```python
from build123d import *

# Parameters (mm, degrees)
BOSS_EXTRUDE1_DEPTH = 30
SKETCH2_R           = 2.25
CUT_EXTRUDE1_DEPTH  = 30
CUT_EXTRUDE2_DEPTH  = 30
CHAMFER1_SIZE       = 5


with BuildPart() as part:
    # Sketch1 → Boss-Extrude1 (new body)
    with BuildSketch(Plane.XY):
        Polygon((0, 22), (0, 0), (45, 0), (45, -3), (-3, -3), (-3, 22), align=None)
    extrude(amount=BOSS_EXTRUDE1_DEPTH)

    # Sketch2 → Cut-Extrude1 (cut)
    with BuildSketch(Plane(origin=(0, 0, 0), x_dir=(0, 0, -1), z_dir=(1, 0, 0))):
        with Locations(Location((-15, 12, 0), (0, 0, 90))):
            Circle(SKETCH2_R)
    extrude(amount=-CUT_EXTRUDE1_DEPTH, mode=Mode.SUBTRACT)

    # Sketch3 → Cut-Extrude2 (cut)
    with BuildSketch(Plane(origin=(0, 0, 0), x_dir=(1, 0, 0), z_dir=(0, 1, 0))):
        with BuildLine():
            Line((7.5, -13.25), (10.5, -13.25))
            ThreePointArc((10.5, -13.25), (12.25, -15), (10.5, -16.75))
            Line((10.5, -16.75), (7.5, -16.75))
            ThreePointArc((7.5, -16.75), (5.75, -15), (7.5, -13.25))
        make_face()
        with BuildLine():
            Line((32.5, -13.25), (35.5, -13.25))
            ThreePointArc((35.5, -13.25), (37.25, -15), (35.5, -16.75))
            Line((35.5, -16.75), (32.5, -16.75))
            ThreePointArc((32.5, -16.75), (30.75, -15), (32.5, -13.25))
        make_face()
    extrude(amount=-CUT_EXTRUDE2_DEPTH, mode=Mode.SUBTRACT)

    # Chamfer1
    chamfer1_edges = [part.edges().sort_by_distance(p)[0] for p in [
        (45, -1.5, 30),
        (-1.5, 22, 30),
        (45, -1.5, 0),
        (-1.5, 22, 0),
    ]]
    chamfer(chamfer1_edges, length=CHAMFER1_SIZE)


solid = part.part
```
Design review of the part built by this model. Coordinates are the model's own, in mm. A direction names the side the tool comes from. Give positions to 0.01 mm unless a question says otherwise; leave off trailing zeros. Loops run counter-clockwise (first coordinate to the right, second up) from the corner with the lowest first, then second, coordinate; pieces in that order, holes last. Notation, with made-up numbers: (4, 25.25) -> (35, 25.25) arc R29 cw to (35, 52.25) -> close; hole circle Ø10 at (6.5, 88.25). An arc over 180 degrees is marked (long way). One line per item, written item: value.
Q1. For pin 1 Ø12 at (x, z) = (24, 4.5) entering from +Y; pin 2 Ø2 at (y, z) = (3.5, 16.5) entering from +X, all flat-tipped, find the tip position at first contact; note any pin that passes through.
Numbers:
pin 1: stops at y = 0
pin 2: stops at x = 0
Q2. Draft analysis for pull direction X (two halves, no side actions). For faces 1 (the flat face through (-2, 19, 28)), 2 (the flat face through (43, -1, 27)), 3 (the flat face through (9, -1, 13.25)), state which applies: pulls with the +X half, pulls with the -X half, needs draft (parallel to the pull), parting line crosses it, or undercut.
Numbers:
face 1: needs draft
face 2: pulls with the +X half
face 3: undercut
Q3. We need section A-A on y = 12. Give the boundary of the cut face in (x, z).
Numbers:
outline: (-3, 0) -> (0, 0) -> (0, 12.75) -> (-3, 12.75) -> close; (-3, 17.25) -> (0, 17.25) -> (0, 30) -> (-3, 30) -> close
Q4. We need section C-C on x = 6.5. Give the boundary of the cut face in (y, z), and give its area (3 significant figures).
Numbers:
outline: (-3, 0) -> (0, 0) -> (0, 13.56) -> (-3, 13.56) -> close; (-3, 16.44) -> (0, 16.44) -> (0, 30) -> (-3, 30) -> close
area: 81.4 mm^2
Q5. Machinability: for faces 4 (the flat face through (22, 0, 15)), 5 (the flat face through (43, -1, 3)), 6 (the flat face through (9, -1, 16.75)), which of the approach directions +Z, -Z, +X, -X, +Y, -Y give a long, thin tool a straight path to every point of the face, cutting with its end or side? Answer none if there is none.
Numbers:
face 4: +Z, -Z, +X, +Y
face 5: -Z, +X, +Y, -Y
face 6: +Y, -Y
Q6. For L1, parallel to Z at x = -1.35, y = 12; L2, parallel to X at y = 3.25, z = 15.5, list the stretches that pass through material, from the lowest coordinate up.
Numbers:
L1: z = 0 to 12.75, 17.25 to 30
L2: x = -3 to 0
Q7. We need section B-B on z = 16. Give the boundary of the cut face in (x, y).
Numbers:
outline: (-3, -3) -> (6.06, -3) -> (6.06, 0) -> (0, 0) -> (0, 9.98) -> (-3, 9.98) -> close; (-3, 14.02) -> (0, 14.02) -> (0, 22) -> (-3, 22) -> close; (11.94, -3) -> (31.06, -3) -> (31.06, 0) -> (11.94, 0) -> close; (36.94, -3) -> (45, -3) -> (45, 0) -> (36.94, 0) -> close
Q8. We need section D-D on z = 11. Give the boundary of the cut face in (x, y).
Numbers:
outline: (-3, -3) -> (45, -3) -> (45, 0) -> (0, 0) -> (0, 22) -> (-3, 22) -> close
